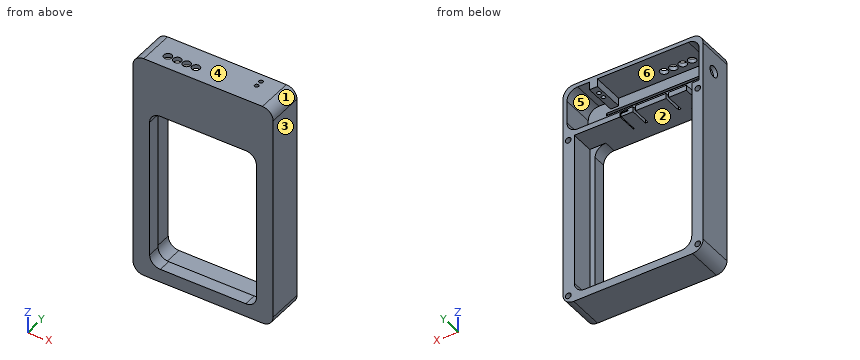
Autodesk Inventor part; units mm, degrees
ref_plane "YZ Plane" through (0, 0, 0) normal (1, 0, 0) x (0, 1, 0)
ref_plane "XZ Plane" through (0, 0, 0) normal (0, 1, 0) x (-1, 0, 0)
ref_plane "XY Plane" through (0, 0, 0) normal (0, 0, 1) x (1, 0, 0)
sketch "Sketch1" plane through (0, 0, 0) normal (0, 1, 0) x (-1, 0, 0)
  line L0 (-52.5, 85) -> (52.5, 85)
  line L1 (52.5, 85) -> (52.5, -85)
  line L2 (52.5, -85) -> (-52.5, -85)
  line L3 (-52.5, -85) -> (-52.5, 85)
  line L4 (-52.5, 85) -> (52.5, -85) construction
  line L5 (52.5, 85) -> (-52.5, -85) construction
  line L6 (40, 45) -> (-40, 45)
  line L7 (-40, 45) -> (-40, -75)
  line L8 (-40, -75) -> (40, -75)
  line L9 (40, -75) -> (40, 45)
  point P0 (0, 0)
  point P1 (0, -75)
  point P2 (0, 0)
  point P3 (0, -85)
  dimension "d0" = 120
  dimension "d1" = 80
  dimension "d2" = 105
  dimension "d3" = 10
  dimension "d4" = 170
extrude "Extrusion1" add sketch "Sketch1" along normal mid plane 27
sketch "Sketch2" plane through (0, 0, 0) normal (0, 1, 0) x (-1, 0, 0)
  line L0 (44, -79) -> (-44, -79)
  line L1 (-44, -79) -> (-44, 45)
  line L2 (-44, 45) -> (44, 45)
  line L3 (44, 45) -> (44, -79)
  line L4 (-40, -75) -> (40, -75)
  line L5 (40, -75) -> (40, 45)
  line L6 (-40, 45) -> (-40, -75)
  point P0 (0, 0)
  dimension "d7" = 4
  dimension "d8" = 4
  dimension "d9" = 4
extrude "Extrusion2" cut sketch "Sketch2" along normal blind 15 and the other way blind 4
sketch "Sketch3" plane through (0, 13.5, 0) normal (0, 1, 0) x (1, 0, 0)
  line L0 (-49.5, -49) -> (49.5, -49)
  line L1 (49.5, -49) -> (49.5, -82)
  line L2 (49.5, -82) -> (-49.5, -82)
  line L3 (-49.5, -82) -> (-49.5, -49)
  line L4 (-52.5, 85) -> (-52.5, -85)
  line L5 (-52.5, -85) -> (52.5, -85)
  line L6 (44, -45) -> (-44, -45)
  point P0 (0, 0)
  point P1 (0, -49)
  dimension "d14" = 3
  dimension "d15" = 3
  dimension "d16" = 4
extrude "Extrusion3" cut sketch "Sketch3" against normal blind 24
sketch "Sketch4" plane through (0, 13.5, 0) normal (0, 1, 0) x (1, 0, 0)
  line L0 (44, -45) -> (-44, -45)
  line L1 (-49.5, -49) -> (49.5, -49)
  line L2 (-44, -45) -> (-40, -45)
  line L3 (-40, -45) -> (-40, -49)
  line L4 (-40, -49) -> (-44, -49)
  line L5 (-44, -49) -> (-44, -45)
  point P0 (0, 0)
  point P1 (-40, 75)
extrude "Extrusion4" cut sketch "Sketch4" against normal up to surface (17.5 mm away)
sketch "Sketch5" plane through (0, 13.5, 0) normal (0, 1, 0) x (1, 0, 0)
  line L0 (44, -45) -> (-40, -45)
  line L1 (-26.6, -48) -> (-24.7, -48)
  line L2 (-24.7, -48) -> (-24.7, -45)
  line L3 (-24.7, -45) -> (-26.6, -45)
  line L4 (-26.6, -45) -> (-26.6, -48)
  line L5 (-1.9, -48) -> (0, -48)
  line L6 (0, -48) -> (0, -45)
  line L7 (0, -45) -> (-1.9, -45)
  line L8 (-1.9, -45) -> (-1.9, -48)
  line L9 (-40, -45) -> (40, -45)
  point P0 (0, 0)
  dimension "d21" = 1.9
  dimension "d22" = 1.9
  dimension "d23" = 22.8
  dimension "d24" = 3
extrude "Extrusion5" cut sketch "Sketch5" against normal blind 14
sketch "Sketch6" plane through (0, 13.5, 0) normal (0, 1, 0) x (1, 0, 0)
  line L0 (-40, -45) -> (40, -45)
  line L1 (9, -45) -> (9, -47.3)
  line L2 (9, -47.3) -> (3.7, -47.3)
  line L3 (3.7, -47.3) -> (3.7, -48)
  line L4 (3.7, -48) -> (9.7, -48)
  line L5 (9.7, -48) -> (9.7, -45)
  line L6 (0, -45) -> (0, -48)
  point P0 (0, 0)
  dimension "d27" = 0.7
  dimension "d28" = 0.7
  dimension "d29" = 3
  dimension "d30" = 6
  dimension "d31" = 9
extrude "Extrusion6" cut sketch "Sketch6" against normal blind 15
fillet "Fillet1" radius 8 12 edges at (-44, 4.75, -79) (44, 4.75, -79) (40, -8.75, -75) (-40, -8.75, -75) (52.5, 0, -85) (-52.5, 0, -85) (-52.5, 0, 85) (-49.5, 1.5, 82) (49.5, 1.5, 82) (52.5, 0, 85) (40, -8.75, 45) (-40, -8.75, 45)
sketch "Sketch7" plane through (0, -10.5, 0) normal (0, 1, 0) x (1, 0, 0)
  line L0 (-36, -74) -> (36, -74)
  line L1 (36, -74) -> (36, -72)
  line L2 (36, -72) -> (-36, -72)
  line L3 (-36, -72) -> (-36, -74)
  line L4 (41.5, -82) -> (-41.5, -82)
  point P0 (0, 0)
  point P1 (0, -72)
  dimension "d35" = 2
  dimension "d36" = 72
  dimension "d37" = 8
extrude "Extrusion7" cut sketch "Sketch7" against normal blind 2
sketch "Sketch8" plane through (-52.5, -13.5, 77) normal (-1, 0, 0) x (0, 0, 1)
  line L0 (0, 0) -> (-154, 0)
  line L1 (-3, 3) -> (-3, 27)
  point P0 (-77, 13.5)
  point P1 (-15, 15)
  dimension "d40" = 15
  dimension "d41" = 12
hole "Hole1" at (-52.5, 1.5, 62) direction (1, 0, 0) diameter 8.4 depth 8 tip angle 118
fillet "Fillet2" radius 8 1 edges at (49.5, 1.5, 49)
sketch "Sketch9" plane through (0, 13.5, 0) normal (0, 1, 0) x (1, 0, 0)
  line L0 (-48.5, 79) -> (48.5, 79) construction
  line L1 (48.5, 79) -> (48.5, -43) construction
  line L2 (48.5, -43) -> (-48.5, -43) construction
  line L3 (-48.5, -43) -> (-48.5, 79) construction
  line L4 (44.5, 85) -> (-44.5, 85)
  line L5 (-52.5, 77) -> (-52.5, -77)
  line L6 (-40, -49) -> (41.5, -49)
  point P0 (0, 0)
  point P1 (0, 79)
  dimension "d50" = 6
  dimension "d51" = 4
  dimension "d52" = 6
hole "Hole2" at (-48.5, 13.5, -79) at (48.5, 13.5, -79) at (48.5, 13.5, 43) at (-48.5, 13.5, 43) direction (0, -1, 0) diameter 4.3 depth 8
sketch "Sketch10" plane through (-44.5, 13.5, 85) normal (0, 0, 1) x (1, 0, 0)
  circle A0 centre (25.3, -16.6) radius 3
  circle A1 centre (32.3, -16.6) radius 3
  circle A2 centre (18.3, -16.6) radius 3
  circle A3 centre (11.3, -16.6) radius 3
  line L0 (-8, 0) -> (-8, -27)
  line L1 (89, -27) -> (0, -27)
  point P0 (44.5, -13.5)
  dimension "d60" = 6
  dimension "d61" = 6
  dimension "d62" = 6
  dimension "d63" = 6
  dimension "d64" = 7
  dimension "d65" = 7
  dimension "d66" = 7
  dimension "d67" = 19.3
  dimension "d68" = 10.4
extrude "Extrusion8" cut sketch "Sketch10" against normal blind 10
sketch "Sketch13" plane through (0, -10.5, 0) normal (0, 1, 0) x (1, 0, 0)
  line L0 (41.5, -82) -> (-41.5, -82)
  line L1 (26.65, -82) -> (32.65, -82)
  line L2 (32.65, -82) -> (32.65, -76)
  line L3 (32.65, -76) -> (26.65, -76)
  line L4 (26.65, -76) -> (26.65, -82)
  point P0 (0, 0)
  point P1 (52.5, -77)
  dimension "d78" = 6
  dimension "d79" = 6
  dimension "d82" = 19.85
extrude "Extrusion10" add sketch "Sketch13" along normal up to surface (24 mm away)
sketch "Sketch11" plane through (-44.5, 13.5, 85) normal (0, 0, 1) x (1, 0, 0)
  circle A0 centre (74.15, -11.19) radius 1.5
  circle A1 centre (74.15, -6.19) radius 1.5
  line L0 (89, -27) -> (0, -27)
  line L1 (97, -27) -> (97, 0)
  point P0 (44.5, -13.5)
  dimension "d71" = 3
  dimension "d72" = 3
  dimension "d73" = 5
  dimension "d76" = 20.81
  dimension "d77" = 22.85
extrude "Extrusion9" cut sketch "Sketch11" against normal blind 10
sketch "Sketch14" plane through (0, 13.5, 0) normal (0, 1, 0) x (1, 0, 0)
  line L0 (-24.7, -48) -> (-26.6, -48)
  line L1 (-40, -49) -> (41.5, -49)
  line L2 (-26.6, -48) -> (-24.7, -48)
  line L3 (-24.7, -48) -> (-24.7, -49)
  line L4 (-24.7, -49) -> (-26.6, -49)
  line L5 (-26.6, -49) -> (-26.6, -48)
  line L6 (0, -48) -> (-1.9, -48)
  line L7 (-1.9, -48) -> (0, -48)
  line L8 (0, -48) -> (0, -49)
  line L9 (0, -49) -> (-1.9, -49)
  line L10 (-1.9, -49) -> (-1.9, -48)
  point P0 (0, 0)
extrude "Extrusion11" cut sketch "Sketch14" against normal blind 2
properties part number "Bottom"
Can you work these out from the model? Positions are in its coordinate system, mm. Face numbers are marked on the shaded views. A direction names the side the tool comes from. Round coordinates to 2 decimals unless told otherwise and drop trailing zeros. Write each loop counter-clockwise with the first axis right and the second up, starting at its lowest first coordinate (ties: lowest second). Pieces come first, ordered by that corner, then holes. Notation, with made-up numbers: M 63.5,89 L 114.5,89 A30 cw 114.5,128 Z; hole C 44,73.5 d6. An arc over 180 degrees is marked long. Use a Markdown table: item, result.
Item 1: I want a section at A-A (z = 22). List the corners of the cut face in (x, y) for me, and give its area (3 significant figures).
Found:
| item | result |
|---|---|
| outline | M -52.5,-13.5 L -40,-13.5 L -40,-4 L -44,-4 L -44,13.5 L -52.5,13.5 Z; M 40,-13.5 L 52.5,-13.5 L 52.5,13.5 L 44,13.5 L 44,-4 L 40,-4 Z |
| area | 535 mm2 |
Item 2: Which directions (+Z, -Z, +X, -X, +Y, -Y) give clear straight access to the entire face, cutting with the end or side of a thin tool? Please do the marked faces 1 and 2.
Found:
| item | result |
|---|---|
| face 1 | +Z, +X, +Y, -Y |
| face 2 | +Y |
Item 3: If I drill on line 1 along X through (y, z) = (7.75, 43); line 2 along Z through (x, y) = (-24.5, -10.75); line 3 along Z through (x, y) = (3.5, 12.75), over which ranges is the centre line in solid material (lowest first)? Write a range as [from, to].
Found:
| item | result |
|---|---|
| line 1 | x = [-52.5, -50.65], [-46.35, -44], [44, 46.35], [50.65, 52.5] |
| line 2 | z = [-85, -75], [45, 72], [74, 85] |
| line 3 | z = [-85, -79], [45, 49], [82, 85] |
Item 4: I want a section at C-C (x = 15). List the corners of the cut face in (y, z) for me.
Found:
| item | result |
|---|---|
| outline | M -13.5,-85 L 13.5,-85 L 13.5,-79 L -4,-79 L -4,-75 L -13.5,-75 Z; M -13.5,45 L 13.5,45 L 13.5,49 L -10.5,49 L -10.5,72 L -12.5,72 L -12.5,74 L -10.5,74 L -10.5,82 L 13.5,82 L 13.5,85 L -13.5,85 Z |
Item 5: I want a section at B-B (x = -19.2). List the corners of the cut face in (y, z) for me.
Found:
| item | result |
|---|---|
| outline | M -13.5,-85 L 13.5,-85 L 13.5,-79 L -4,-79 L -4,-75 L -13.5,-75 Z; M -13.5,45 L 13.5,45 L 13.5,49 L -10.5,49 L -10.5,72 L -12.5,72 L -12.5,74 L -10.5,74 L -10.5,82 L -6.1,82 L -6.1,85 L -13.5,85 Z; M -0.1,82 L 13.5,82 L 13.5,85 L -0.1,85 Z |
Item 6: I want a section at D-D (z = 62). List the corners of the cut face in (x, y) for me.
Found:
| item | result |
|---|---|
| outline | M -52.5,-13.5 L 52.5,-13.5 L 52.5,13.5 L 49.5,13.5 L 49.5,-10.5 L -49.5,-10.5 L -49.5,-2.7 L -52.5,-2.7 Z; M -52.5,5.7 L -49.5,5.7 L -49.5,13.5 L -52.5,13.5 Z |
Item 7: We'd pull the mould along X, two halves only. Please class the marked faces 3, 4, 5 and 6: released by +X, released by -X, zero draft, split by the parting line, or undercut.
Found:
| item | result |
|---|---|
| face 3 | released by +X |
| face 4 | zero draft |
| face 5 | undercut |
| face 6 | undercut |
